```python
from build123d import *

# Parameters (mm, degrees)
F1_DEPTH    = 10
F2_R        = 3
F3_DEPTH    = 25
F4_R        = 4.99999
F5_T1_DEPTH = 10


# Not quite as in the source:
# - a fillet or chamfer that OpenCascade refuses, or shapes differently, is made with other operations: its cross-section is extruded or revolved along the edge and cut away or added
# - a fillet or chamfer is up to 0.001 mm smaller than in the source, because OpenCascade refuses the exact size


with BuildPart() as f1:
    # F0 (on Right) → F1 (new body)
    with BuildSketch(Plane.YZ):
        Polygon((-20.7655076647, 0), (0, 0), (2.7424137787, 4.75), (0, 9.5), (-5.4848275573, 9.5), (-8.3715789032, 4.5), (-8.3715789032, 3), (-20.7655076647, 3), align=None)
        Polygon((-4.3301270189, 2), (-5.9178402592, 4.75), (-4.3301270189, 7.5), (-1.1547005384, 7.5), (0.4330127019, 4.75), (-1.1547005384, 2), align=None, mode=Mode.SUBTRACT)
    extrude(amount=F1_DEPTH)

    # F2 (on face) → F3 (cut)
    with BuildSketch(Plane.XY.offset(3)):
        with Locations((5, -16.0806495696)):
            Circle(F2_R)
    extrude(amount=-F3_DEPTH, mode=Mode.SUBTRACT)

    # F4 (radius 5 in the source; OpenCascade refuses exactly that, so slightly less here)
    f4_edges = [f1.edges().sort_by_distance(p)[0] for p in [
        (0, -20.765508, 1.5),
        (10, -20.765508, 1.5),
    ]]
    fillet(f4_edges, radius=F4_R)

    # F5: fillet of radius 3 on 1 edges, made by hand

    # F5_s2 → F5_t1 (join)
    with BuildSketch(Plane.YZ):
        with BuildLine():
            ThreePointArc((-10.9696551146, 3), (-9.4696551146, 3.4019237886), (-8.3715789032, 4.5))
            Line((-8.3715789032, 4.5), (-8.3715789032, 3))
            Line((-8.3715789032, 3), (-10.9696551146, 3))
        make_face()
    extrude(amount=F5_T1_DEPTH)


solid = f1.part
```
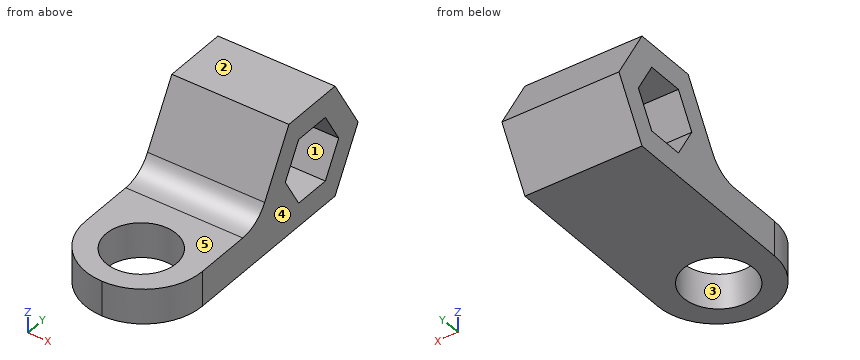
Part model, mm, in its own coordinate system. Face numbers are marked on the shaded views. A direction names the side the tool comes from. Give positions to 0.01 mm unless a question says otherwise; leave off trailing zeros. Order: outer loops, then holes, each group sorted by start corner. A loop starts at its lowest first (then second) coordinate and runs counter-clockwise, first axis right, second up. Notation, with made-up numbers: M 18,37 L 57,37 A17 ccw 57,46 Z; hole C 26,77.5 d7. An arc over 180 degrees is marked long. Use a Markdown table: item, result. Add a question column.
(1) Probe line 1 along Y through (x, z) = (5, 2.15); line 2 along Y through (x, z) = (4.75, 3.75); line 3 along X through (y, z) = (-13.75, 2). List the from-to ranges inside material, lowest first. Write a range as [from, to].
(2) Saw through at B-B, the plane x = 4.75. Give the cut face in (y, z).
(3) 3-axis set-ups, long thin cutter, end or side, ignore diameter. For the marked faces 1 and 2: which of +Z, -Z, +X, -X, +Y, -Y reach the whole face in a straight line?
(4) Saw through at D-D, the plane z = 4. Give the cut face in (x, y), and give its area (3 significant figures).
(5) Drop flat-ended pins along their axis: P1, Ø4, axis at x = 6.5, z = 7, coming from the -Y side; P2, Ø3.5, axis at x = 5, y = -16.08, coming from the +Z side; P3, Ø3, axis at x = 5.5, y = -14, coming from the +Z side; P4, Ø1.5, axis at x = 1, z = 3.5, coming from the -Y side. Give the stop position or say it passes through.
(6) Mould opens along X. For the marked faces 3, 4 and 5 say: +X half, -X half, draft (parallel to the pull), parting line (faces both ways), or undercut.
(7) Saw through at A-A, the plane y = -2. Give the cut face in (x, z).
(8) Saw through at C-C, the plane z = 2.25. Give the number of separate pieces and of enclosed holes in the cut face, and give its area (3 significant figures).
Answer key:
| question | item | result |
|---|---|---|
| 1 | line 1 | [-20.77, -19.08], [-13.08, -4.42], [-1.07, 1.24] |
| 1 | line 2 | [-8.99, -5.34], [-0.14, 2.17] |
| 1 | line 3 | [0, 3.11], [6.89, 10] |
| 2 | outline | M -20.76,0 L -19.07,0 L -19.07,3 L -20.76,3 Z; M -13.09,0 L 0,0 L 2.74,4.75 L 0,9.5 L -5.48,9.5 L -8.37,4.5 A3 cw -10.97,3 L -13.09,3 Z; hole M -5.92,4.75 L -4.33,2 L -1.15,2 L 0.43,4.75 L -1.15,7.5 L -4.33,7.5 Z |
| 3 | face 1 | +X, -X |
| 3 | face 2 | +Z, +X, -X, +Y, -Y |
| 4 | outline | M 0,-8.73 L 10,-8.73 L 10,-5.48 L 0,-5.48 Z; M 0,0 L 10,0 L 10,2.31 L 0,2.31 Z |
| 4 | area | 55.6 mm^2 |
| 5 | P1 | y = -8.08 |
| 5 | P2 | through |
| 5 | P3 | z = 3 |
| 5 | P4 | y = -19.39 |
| 6 | face 3 | undercut |
| 6 | face 4 | +X half |
| 6 | face 5 | draft |
| 7 | outline | M 0,0 L 10,0 L 10,2 L 0,2 Z; M 0,7.5 L 10,7.5 L 10,9.5 L 0,9.5 Z |
| 8 | separate pieces | 2 |
| 8 | enclosed holes | 1 |
| 8 | area | 147 mm^2 |
